Part model, mm, in its own coordinate system. A direction names the side the tool comes from. Coordinates: 2 decimals unless noted, no trailing zeros. Write each loop counter-clockwise with the first axis right and the second up, starting at its lowest first coordinate (ties: lowest second). Pieces come first, ordered by that corner, then holes. Notation, with made-up numbers: (0, -0.75) -> (31, -0.75) arc R33 ccw to (31, 27.25) -> close; hole circle Ø5 at (55.5, 88). An arc over 180 degrees is marked (long way). Write item = value, one per line. Start each with the question number.
Q1. Pull direction Z, two halves, no side cores. Call faces 1 (the cylindrical face through (-19.527, 0.07, -148.724)), 2 (the flat face through (120, 5, -31)), 3 (the cylindrical face through (-107.53, 4.51, 82.45)): released by +Z, released by -Z, zero draft, split by the parting line, or undercut.
Q2. Pin check, flat tip, straight feed: P1, Ø2, axis at y = 0, z = 73.5, coming from the +X side. Stop position of the tip, or through.
Q3. Probe line 1 (Z direction, x = 0, y = -4.3); line 2 (Z direction, x = 0, y = 0.25). List the from-to ranges inside material, lowest first.
Q4. Tool access for faces 4 (the cylindrical face through (129.958, -4.507, -40.926)), 5 (the flat face through (120, -5, -31)), 6 (the cylindrical face through (129.958, 4.507, -40.926)): list every direction of +Z, -Z, +X, -X, +Y, -Y with a clear straight run to the whole face (end or side of a thin tool).
Q5. Band-saw the part on B-B, the plane x = 0. List the corners of the cut face in (y, z).
Q6. Band-saw the part on C-C, the plane y = 1. List the corners of the cut face in (x, z), plus the area to 3 significant figures.
Q7. Band-saw the part on A-A, the plane z = 0. List the corners of the cut face in (x, y).
from build123d import *

# Parameters (mm, degrees)
SKETCH1_R           = 150
SKETCH1_R_2         = 123.5
BOSS_EXTRUDE1_DEPTH = 5
SKETCH2_R           = 136.25
SKETCH2_R_2         = 135.5
CUT_EXTRUDE1_DEPTH  = 1


with BuildPart() as part:
    # Sketch1 → Boss-Extrude1 (new body, symmetric)
    with BuildSketch(Plane(origin=(0, 0, 0), x_dir=(1, 0, 0), z_dir=(0, 1, 0))):
        Circle(SKETCH1_R)
        Circle(SKETCH1_R_2, mode=Mode.SUBTRACT)
    extrude(amount=BOSS_EXTRUDE1_DEPTH, both=True)

    # Sketch2 → Cut-Extrude1 (cut)
    with BuildSketch(Plane(origin=(0, 5, 0), x_dir=(1, 0, 0), z_dir=(0, 1, 0))):
        Circle(SKETCH2_R)
        Circle(SKETCH2_R_2, mode=Mode.SUBTRACT)
    cut_extrude1 = extrude(amount=-CUT_EXTRUDE1_DEPTH, mode=Mode.SUBTRACT)

    # Mirror1: Cut-Extrude1 across plane
    add(cut_extrude1.mirror(Plane.ZX), mode=Mode.SUBTRACT)


solid = part.part
Ans:
q1.face_1 = split by the parting line
q1.face_2 = zero draft
q1.face_3 = undercut
q2.P1 = 131.32
q3.line_1 = -150 to -136.25, -135.5 to -123.5, 123.5 to 135.5, 136.25 to 150
q3.line_2 = -150 to -123.5, 123.5 to 150
q4.face_4 = -Y
q4.face_5 = +Z, -Z, +X, -X, -Y
q4.face_6 = +Y
q5.outline = (-5, -150) -> (5, -150) -> (5, -136.25) -> (4, -136.25) -> (4, -135.5) -> (5, -135.5) -> (5, -123.5) -> (-5, -123.5) -> (-5, -135.5) -> (-4, -135.5) -> (-4, -136.25) -> (-5, -136.25) -> close; (-5, 123.5) -> (5, 123.5) -> (5, 135.5) -> (4, 135.5) -> (4, 136.25) -> (5, 136.25) -> (5, 150) -> (-5, 150) -> (-5, 136.25) -> (-4, 136.25) -> (-4, 135.5) -> (-5, 135.5) -> close
q6.outline = circle Ø300 at (0, 0); hole circle Ø247 at (0, 0)
q6.area = 22,800 mm2
q7.outline = (-150, -5) -> (-136.25, -5) -> (-136.25, -4) -> (-135.5, -4) -> (-135.5, -5) -> (-123.5, -5) -> (-123.5, 5) -> (-135.5, 5) -> (-135.5, 4) -> (-136.25, 4) -> (-136.25, 5) -> (-150, 5) -> close; (123.5, -5) -> (135.5, -5) -> (135.5, -4) -> (136.25, -4) -> (136.25, -5) -> (150, -5) -> (150, 5) -> (136.25, 5) -> (136.25, 4) -> (135.5, 4) -> (135.5, 5) -> (123.5, 5) -> close
